Print and shaded views of the part. All mm, measured from the part's lowest x, y and z. A direction names the side the tool comes from. Round coordinates to 2 decimals unless told otherwise and drop trailing zeros. Loops run counter-clockwise (first coordinate to the right, second up) from the corner with the lowest first, then second, coordinate; pieces in that order, holes last. Notation, with made-up numbers: (87.5, 37) - (142.5, 37) arc R29 ccw to (142.5, 74) - close; hole circle Ø4 at (83, 82). An arc over 180 degrees is marked (long way). Answer as a JSON object with one key per item and string values.
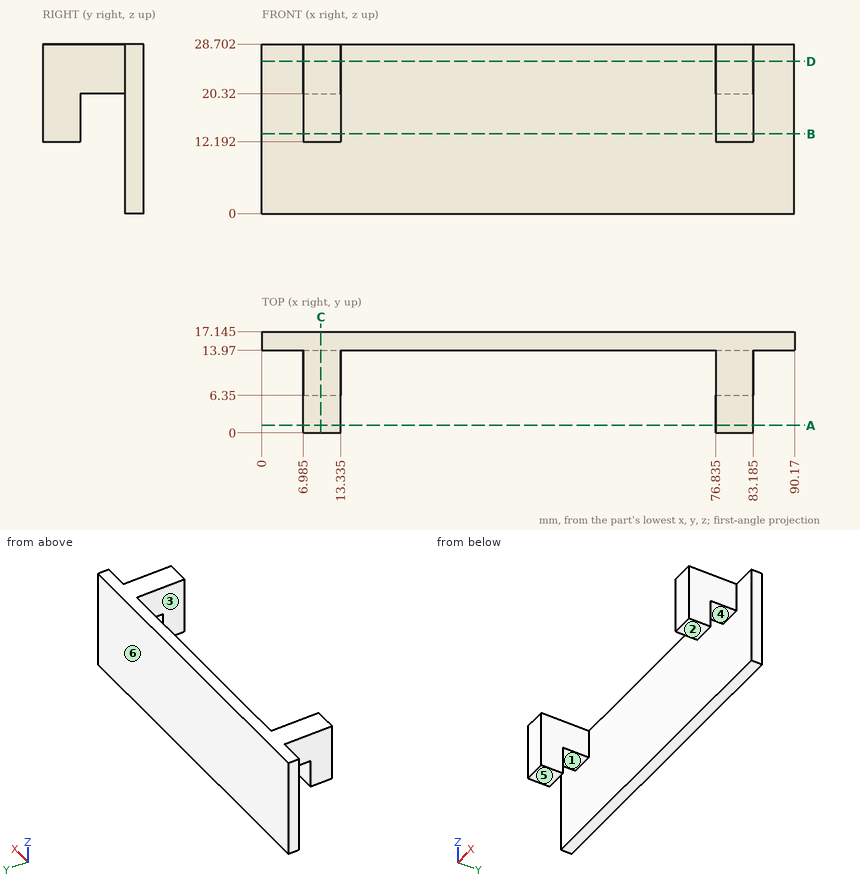
1) Two-plate mould, pull along Y, no slides. Class the marked faces 4, 5 and 6: pulls with the +Y half, pulls with the -Y half, needs draft (parallel to the pull), parting line crosses it, or undercut.
Values follow:
{"face 4": "undercut", "face 5": "needs draft", "face 6": "pulls with the +Y half"}
2) Slice it at D-D on z = 25.75. List the corners of the cut face in (x, y) (3 decimals).
Values follow:
{"outline": "(0, 13.97) - (6.985, 13.97) - (6.985, 0) - (13.335, 0) - (13.335, 13.97) - (76.835, 13.97) - (76.835, 0) - (83.185, 0) - (83.185, 13.97) - (90.17, 13.97) - (90.17, 17.145) - (0, 17.145) - close"}
3) Slice it at A-A on y = 1.25. List the corners of the cut face in (x, z) (3 decimals).
Values follow:
{"outline": "(6.985, 12.192) - (13.335, 12.192) - (13.335, 28.702) - (6.985, 28.702) - close; (76.835, 12.192) - (83.185, 12.192) - (83.185, 28.702) - (76.835, 28.702) - close"}
4) Slice it at B-B on z = 13.5. List the corners of the cut face in (x, y) (3 decimals).
Values follow:
{"outline": "(0, 13.97) - (90.17, 13.97) - (90.17, 17.145) - (0, 17.145) - close; (6.985, 0) - (13.335, 0) - (13.335, 6.35) - (6.985, 6.35) - close; (76.835, 0) - (83.185, 0) - (83.185, 6.35) - (76.835, 6.35) - close"}
5) Probe probe 1 along X at (y, z) = (12.75, 23.75) (3 decimals); probe 2 along Y at (x, z) = (10.5, 16.25) (3 decimals); probe 3 along Y at (x, z) = (31, 12.25) (3 decimals). List the from-to ranges inside material, lowest first.
Values follow:
{"probe 1": "6.985 to 13.335, 76.835 to 83.185", "probe 2": "0 to 6.35, 13.97 to 17.145", "probe 3": "13.97 to 17.145"}
6) Slice it at C-C on x = 10. List the corners of the cut face in (y, z) (3 decimals).
Values follow:
{"outline": "(0, 12.192) - (6.35, 12.192) - (6.35, 20.32) - (13.97, 20.32) - (13.97, 0) - (17.145, 0) - (17.145, 28.702) - (0, 28.702) - close"}
7) Tool access for the marked faces 1, 2 and 3: list every direction of +Z, -Z, +X, -X, +Y, -Y with a clear straight run to the whole face (end or side of a thin tool).
Values follow:
{"face 1": "-Z, +X, -X", "face 2": "-Z, +X, -X, -Y", "face 3": "+Z, -Z, -Y"}
8) Drop flat-ended pins along their axis: P1, Ø1.9, axis at x = 80, y = 11.5, coming from the -Z side; P2, Ø8, axis at x = 53.5, z = 6.5, coming from the -Y side; P3, Ø4, axis at y = 7.5, z = 22.5, coming from the -X side (3 decimals). Give the stop position or say it passes through.
Values follow:
{"P1": "z = 20.32", "P2": "y = 13.97", "P3": "x = 6.985"}
